Check sheet for the modelled part. Datum: model origin and axes. Units: mm. A direction names the side the tool comes from. Round coordinates to 2 decimals unless told otherwise and drop trailing zeros. Order: outer loops, then holes, each group sorted by start corner. A loop starts at its lowest first (then second) coordinate and runs counter-clockwise, first axis right, second up. Notation, with made-up numbers: (-19, -18.75) -> (-12, -18.75) arc R30 cw to (-12, 9.25) -> close; hole circle Ø11 at (61.5, 80). An arc over 180 degrees is marked (long way). Answer in a Markdown table with one row per item.
from build123d import *

# Parameters (mm, degrees)
SKETCH2_W           = 93.98
SKETCH2_H           = 55.88
BOSS_EXTRUDE1_DEPTH = 12.7
SKETCH3_W           = 33.02
SKETCH3_H           = 30.48
BOSS_EXTRUDE2_DEPTH = 17.78
FILLET1_R           = 2.54
SKETCH4_R           = 10.795
CUT_EXTRUDE1_DEPTH  = 25.4
CUT_EXTRUDE2_START  = -25.4
SKETCH5_R           = 10.795
CUT_EXTRUDE2_DEPTH  = 25.4
FILLET2_R           = 2.54
FILLET3_R           = 15.24


with BuildPart() as part:
    # Sketch2 → Boss-Extrude1 (new body)
    with BuildSketch(Plane(origin=(0, 0, 0), x_dir=(1, 0, 0), z_dir=(0, 1, 0))):
        with BuildLine():
            ThreePointArc((-93.688069253, -11.244332686), (-70.349230661, -12.298232488), (-46.99, -12.696270789))
            ThreePointArc((-46.99, -12.696270789), (-23.630769339, -12.298232488), (-0.291930747, -11.244332686))
            ThreePointArc((-0.291930747, -11.244332686), (8.940138318, -6.930983214), (12.7, 2.54))
            Line((12.7, 2.54), (12.7, 12.7))
            Line((12.7, 12.7), (50.8, 12.7))
            Line((50.8, 12.7), (50.8, 43.18))
            Line((50.8, 43.18), (12.7, 43.18))
            Line((12.7, 43.18), (12.7, 53.34))
            ThreePointArc((12.7, 53.34), (8.940138318, 62.810983214), (-0.291930747, 67.124332686))
            ThreePointArc((-0.291930747, 67.124332686), (-23.630769339, 68.178232488), (-46.99, 68.576270789))
            ThreePointArc((-46.99, 68.576270789), (-70.349230661, 68.178232488), (-93.688069253, 67.124332686))
            ThreePointArc((-93.688069253, 67.124332686), (-102.920138318, 62.810983214), (-106.68, 53.34))
            Line((-106.68, 53.34), (-106.68, 43.18))
            Line((-106.68, 43.18), (-144.78, 43.18))
            Line((-144.78, 43.18), (-144.78, 12.7))
            Line((-144.78, 12.7), (-106.68, 12.7))
            Line((-106.68, 12.7), (-106.68, 2.54))
            ThreePointArc((-106.68, 2.54), (-102.920138318, -6.930983214), (-93.688069253, -11.244332686))
        make_face()
        with Locations((-46.99, 27.94)):
            Rectangle(SKETCH2_W, SKETCH2_H, mode=Mode.SUBTRACT)
    extrude(amount=BOSS_EXTRUDE1_DEPTH)

    # Sketch3 → Boss-Extrude2 (add)
    with BuildSketch(Plane(origin=(0, 12.7, 0), x_dir=(1, 0, 0), z_dir=(0, 1, 0))):
        with Locations((34.29, 27.94)):
            Rectangle(SKETCH3_W, SKETCH3_H)
        with Locations((-128.27, 27.94)):
            Rectangle(SKETCH3_W, SKETCH3_H)
    extrude(amount=BOSS_EXTRUDE2_DEPTH)

    # Fillet1
    fillet1_edges = [part.edges().sort_by_distance(p)[0] for p in [
        (17.78, 12.7, -27.94),
        (-111.76, 12.7, -27.94),
    ]]
    fillet(fillet1_edges, radius=FILLET1_R)

    # Sketch4 → Cut-Extrude1 (cut)
    with BuildSketch(Plane(origin=(50.8, 0, 0), x_dir=(0, 0, -1), z_dir=(1, 0, 0))):
        with Locations((27.94, 15.24)):
            Circle(SKETCH4_R)
    extrude(amount=-CUT_EXTRUDE1_DEPTH, mode=Mode.SUBTRACT)

    # Sketch5 → Cut-Extrude2 (cut)
    with BuildSketch(Plane.ZY.offset(144.78).offset(CUT_EXTRUDE2_START)):
        with Locations(Location((-27.94, 15.24, 0), (0, 0, 180))):
            Circle(SKETCH5_R)
    extrude(amount=CUT_EXTRUDE2_DEPTH, mode=Mode.SUBTRACT)

    # Fillet2
    fillet2_edges = [part.edges().sort_by_distance(p)[0] for p in [
        (12.7, 6.35, -43.18),
        (12.7, 6.35, -12.7),
        (-106.68, 6.35, -43.18),
        (-106.68, 6.35, -12.7),
    ]]
    fillet(fillet2_edges, radius=FILLET2_R)

    # Fillet3
    fillet3_edges = [part.edges().sort_by_distance(p)[0] for p in [
        (34.29, 30.48, -43.18),
        (34.29, 30.48, -12.7),
        (-128.27, 30.48, -43.18),
        (-128.27, 30.48, -12.7),
    ]]
    fillet(fillet3_edges, radius=FILLET3_R - 0.0001)  # a hair under: the kernel refuses the full size


solid = part.part
Item 1: Set-up check for faces 4 (the flat face through (17.78, 21, -28)), 5 (the flat face through (-48, 6, -55.88)), 6 (the flat face through (-127, 8, -12.7)): record each of +Z, -Z, +X, -X, +Y, -Y from which the full face is reachable in a straight line by a thin tool's end or side.
Result sheet:
| item | result |
|---|---|
| face 4 | +Z, -Z, +Y |
| face 5 | +Y, -Y |
| face 6 | +Z, -X, +Y, -Y |
Item 2: Cross-section at C-C (x = -77.5). Record the boundary of the cut face in (y, z), and give its area (3 significant figures).
Result sheet:
| item | result |
|---|---|
| outline | (0, -67.93) -> (12.7, -67.93) -> (12.7, -55.88) -> (0, -55.88) -> close; (0, 0) -> (12.7, 0) -> (12.7, 12.05) -> (0, 12.05) -> close |
| area | 306 mm^2 |
Item 3: Cross-section at A-A (z = -6). Record the boundary of the cut face in (x, y), and give its area (3 significant figures).
Result sheet:
| item | result |
|---|---|
| outline | (-106.68, 0) -> (-93.98, 0) -> (-93.98, 12.7) -> (-106.68, 12.7) -> close; (0, 0) -> (12.7, 0) -> (12.7, 12.7) -> (0, 12.7) -> close |
| area | 323 mm^2 |
Item 4: Scan lines: line 1 (X direction, y = 9.5, z = -9.5); line 2 (X direction, y = 8, z = -14.5); line 3 (Y direction, x = 38, z = -27). Record each from-to range of solid material in increasing order. Write a range as [from, to].
Result sheet:
| item | result |
|---|---|
| line 1 | x = [-106.68, -93.98], [0, 12.7] |
| line 2 | x = [-144.78, -93.98], [0, 50.8] |
| line 3 | y = [0, 4.49], [25.99, 30.45] |
Item 5: Mould release check, pull along Z, two halves, no side actions. Record for faces 1 (the cylindrical face through (-70.02, 6.26, -68.19)), 2 (the cylindrical face through (8.839, 6.261, 7.037)), 3 (the flat face through (0, 6, -28)): pulls with the +Z half, pulls with the -Z half, needs draft (parallel to the pull), parting line crosses it, or undercut.
Result sheet:
| item | result |
|---|---|
| face 1 | pulls with the -Z half |
| face 2 | pulls with the +Z half |
| face 3 | undercut |
Item 6: Depth check by flat-ended pin: P1, Ø4.5, axis at x = 25, y = 10, coming from the -Z side; P2, Ø10, axis at x = -61.5, y = 5, coming from the -Z side; P3, Ø8, axis at x = 30, y = 21, coming from the +Z side. Enter the tip coordinate at first touch or a pass-through.
Result sheet:
| item | result |
|---|---|
| P1 | stops at z = -43.18 |
| P2 | stops at z = -68.49 |
| P3 | stops at z = -12.8 |
